Autodesk Inventor part; units mm, degrees
ref_plane "Work Plane1" through (1.8331, 3.175, -114.3) normal (-0.8660254, 0.5, 0) x (0, 0, 1)
ref_plane "Work Plane2" through (-3.6662, -6.35, 0) normal (0, 0, 1) x (1, 0, 0)
ref_plane "YZ Plane" through (0, 0, 0) normal (1, 0, 0) x (0, 1, 0)
sketch "Sketch1" plane through (0, 0, 0) normal (0, 0, 1) x (1, 0, 0)
  line L0 (7.3323, 0) -> (3.6662, -6.35)
  line L1 (3.6662, -6.35) -> (-3.6662, -6.35)
  line L2 (-3.6662, -6.35) -> (-7.3323, 0)
  line L3 (-7.3323, 0) -> (-3.6662, 6.35)
  line L4 (-3.6662, 6.35) -> (3.6662, 6.35)
  line L5 (3.6662, 6.35) -> (7.3323, 0)
  point P0 (0, 0)
  point P1 (0, 0)
  dimension "d0" = 12.7
extrude "Extrusion1" add sketch "Sketch1" along normal blind 114.3
sketch "Sketch2" plane through (0, 0, 114.3) normal (0, 0, 1) x (1, 0, 0)
  circle A0 centre (0, 0) radius 4.7625
  dimension "d3" = 9.525
extrude "Extrusion2" add sketch "Sketch2" along normal blind 25.4
mirror "Mirror1" about plane through (0, 0, 0) normal (0, 0, -1) of "Extrusion2", "Extrusion1"
ref_plane "Work Plane1" through (1.8331, 3.175, -114.3) normal (-0.8660254, 0.5, 0) x (0, 0, 1)
sketch "Sketch3" plane through (1.8331, 3.175, -114.3) normal (-0.8660254, 0.5, 0) x (0, 0, 1)
  line L0 (-25.4, 1.0963) -> (-25.4, -8.4287) construction
  line L1 (0, 1.0963) -> (0, -8.4287) construction
  line L2 (-25.4, 1.0963) -> (0, 1.0963) construction
  line L3 (-25.4, -8.4287) -> (0, -8.4287) construction
  line L4 (228.6, 3.6662) -> (0, 3.6662) construction
  line L5 (228.6, -7.3323) -> (228.6, 0) construction
  line L6 (228.6, 0) -> (0, 0) construction
  line L7 (0, -7.3323) -> (0, 0) construction
  line L8 (228.6, -7.3323) -> (0, -7.3323) construction
  line L9 (228.6, 0) -> (228.6, 3.6662) construction
  line L10 (228.6, 3.6662) -> (0, 3.6662) construction
  line L11 (0, 0) -> (0, 3.6662) construction
  line L12 (228.6, 0) -> (0, 0) construction
  line L13 (228.6, -10.9985) -> (228.6, -7.3323) construction
  line L14 (228.6, -7.3323) -> (0, -7.3323) construction
  line L15 (0, -10.9985) -> (0, -7.3323) construction
  line L16 (228.6, -10.9985) -> (0, -10.9985) construction
  line L17 (254, 1.0963) -> (254, -8.4287) construction
  line L18 (228.6, 1.0963) -> (228.6, -8.4287) construction
  line L19 (228.6, 1.0963) -> (254, 1.0963) construction
  line L20 (228.6, -8.4287) -> (254, -8.4287) construction
  line L21 (-25.4, -3.6662) -> (254, -3.6662) construction
  line L22 (3.81, 14.6218) -> (3.81, 1.9218)
  line L23 (3.81, 1.9218) -> (5.334, 1.9218)
  line L24 (5.334, 1.9218) -> (5.334, 14.6218)
  line L25 (5.334, 14.6218) -> (3.81, 14.6218)
  line L26 (19.6342, 14.6218) -> (19.6342, 1.9218)
  line L27 (19.6342, 1.9218) -> (21.1582, 1.9218)
  line L28 (21.1582, 1.9218) -> (21.1582, 14.6218)
  line L29 (21.1582, 14.6218) -> (19.6342, 14.6218)
  line L30 (0, 1.9218) -> (228.6, 1.9218) construction
  line L31 (51.054, 1.9218) -> (51.054, 14.6218)
  line L32 (51.054, 14.6218) -> (52.578, 14.6218)
  line L33 (52.578, 14.6218) -> (52.578, 1.9218)
  line L34 (51.054, 1.9218) -> (52.578, 1.9218)
  line L35 (176.022, 1.9218) -> (176.022, 14.6218)
  line L36 (176.022, 14.6218) -> (177.546, 14.6218)
  line L37 (177.546, 14.6218) -> (177.546, 1.9218)
  line L38 (176.022, 1.9218) -> (177.546, 1.9218)
  line L39 (0, 13.7963) -> (0, 1.0963)
  line L40 (0, 1.0963) -> (1.6002, 1.0963)
  line L41 (1.6002, 1.0963) -> (1.6002, 13.7963)
  line L42 (1.6002, 13.7963) -> (0, 13.7963)
  line L43 (228.346, 13.7963) -> (228.346, 1.0963)
  line L44 (228.346, 1.0963) -> (228.6, 1.0963)
  line L45 (228.6, 1.0963) -> (228.6, 13.7963)
  line L46 (228.6, 13.7963) -> (228.346, 13.7963)
  point P0 (114.3, -3.6662)
  dimension "d6" = 12.7
  dimension "d7" = 1.524
  dimension "d10" = 1.524
  dimension "d11" = 5.588
  dimension "d13" = 1.524
  dimension "d14" = 1.524
  dimension "d16" = 14.3002
  dimension "d18" = 123.444
  dimension "d19" = 61.722
  dimension "d23" = 1.6002
  dimension "d24" = 12.7
  dimension "d25" = 12.7
  dimension "d26" = 0.254
  dimension "d27" = 3.81
revolve "Revolution1" cut sketch "Sketch3" angle 360 about axis through (0, 0, -139.7) along (0, 0, 1)
ref_plane "Work Plane2" through (-3.6662, -6.35, 0) normal (0, 0, 1) x (1, 0, 0)
equation "\"d10\" = d7"
equation "\"d13\" = d7"
equation "\"d14\" = d7"
equation "\"d25\" = d6"
properties part number "0.5 in Hex Shaft V3" material "Steel"
Design review of the part built by this model. Coordinates are the model's own, in mm. A direction names the side the tool comes from. Give positions to 0.01 mm unless a question says otherwise; leave off trailing zeros. Write each loop counter-clockwise with the first axis right and the second up, starting at its lowest first coordinate (ties: lowest second). Pieces come first, ordered by that corner, then holes. Notation, with made-up numbers: (-4.75, -37) -> (21.25, -37) arc R16 cw to (21.25, -29) -> close; hole circle Ø11 at (61, 54). An arc over 180 degrees is marked (long way). Answer in a Markdown table with one row per item.
(1) Clearance check with flat-ended pins moving along their axes: pin 1 (1.5 mm diameter, centred on y = -3.5, z = 95, fed in from -X); pin 2 (4 mm diameter, centred on y = -5, z = -48, fed in from +X); pin 3 (1 mm diameter, centred on y = 2, z = 39.5, fed in from +X). State where each tip first meets the part, or that it passes through.
Results:
| item | result |
|---|---|
| pin 1 | x = -5.74 |
| pin 2 | x = 5.6 |
| pin 3 | x = 6.47 |
(2) Consider section A-A (z = -32). State the section outline as (x, y) points, then the cut area to 3 significant figures.
Results:
| item | result |
|---|---|
| outline | (-7.33, 0) -> (-3.67, -6.35) -> (3.67, -6.35) -> (7.33, 0) -> (3.67, 6.35) -> (-3.67, 6.35) -> close |
| area | 140 mm2 |
(3) For faces 5 (the cylindrical face through (4.434, 3.4, -109.717)), 6 (the flat face through (4, 3, -112.7)), 7 (the cylindrical face through (-3.78, 2.9, 126.82)), list the 3-axis set-ups (+Z, -Z, +X, -X, +Y, -Y) from which the entire face can be reached by the end or side of a thin tool; tool diameter is ignored.
Results:
| item | result |
|---|---|
| face 5 | none |
| face 6 | -Z |
| face 7 | +Z |
(4) Mouldability with a two-part tool opening along Z and no side actions: class faces 1 (the flat face through (0, 0, -139.7)), 2 (the flat face through (0, 6, -63.246)), 3 (the cylindrical face through (4.434, 3.4, -93.893)), 4 (the flat face through (-5.525, -3.131, 89.002)) as +Z half, -Z half, draft (parallel to the pull), parting line (faces both ways), or undercut.
Results:
| item | result |
|---|---|
| face 1 | -Z half |
| face 2 | undercut |
| face 3 | undercut |
| face 4 | draft |
(5) To check wall thickness, follow probe 1 along Z at (x, y) = (5.25, -3); probe 2 along Y at (x, z) = (0, -120.5); probe 3 along Z at (x, y) = (-3.75, -3.25). State the ranges of each line that lie inside material, in increasing order.
Results:
| item | result |
|---|---|
| probe 1 | -112.7 to -110.49, -108.97 to -94.67, -93.14 to -63.25, -61.72 to 61.72, 63.25 to 114.05 |
| probe 2 | -4.76 to 4.76 |
| probe 3 | -112.7 to 114.05 |
